Autodesk Inventor part; units mm, degrees
ref_plane "YZ Plane" through (0, 0, 0) normal (1, 0, 0) x (0, 1, 0)
ref_plane "XZ Plane" through (0, 0, 0) normal (0, 1, 0) x (-1, 0, 0)
ref_plane "XY Plane" through (0, 0, 0) normal (0, 0, 1) x (1, 0, 0)
sketch "스케치1" plane through (0, 0, 0) normal (0, 0, 1) x (1, 0, 0)
  line L0 (-103.5, -63) -> (-103.5, 58)
  line L1 (-98.5, -63) -> (-103.5, -63)
  line L2 (-98.5, 58) -> (-98.5, -63)
  line L3 (98.5, 58) -> (-98.5, 58)
  line L4 (98.5, -63) -> (98.5, 58)
  line L5 (103.5, -63) -> (98.5, -63)
  line L6 (103.5, 58) -> (103.5, -63)
  arc A0 (103.5, 58) -> (98.5, 63) centre (98.5, 58) ccw
  line L7 (-98.5, 63) -> (98.5, 63)
  arc A1 (-98.5, 63) -> (-103.5, 58) centre (-98.5, 58) ccw
  line L8 (-98.5, -63) -> (98.5, -63)
  point P0 (0, 0)
extrude "돌출1" add sketch "스케치1" along normal blind 5
sketch "스케치2" plane through (0, 0, 5) normal (0, 0, 1) x (1, 0, 0)
  line L0 (-91.5, 58) -> (91.5, 58)
  line L1 (98.5, 51) -> (98.5, -46)
  line L2 (91.5, -53) -> (-91.5, -53)
  line L3 (-98.5, -46) -> (-98.5, 51)
  line L4 (98.5, 63) -> (-98.5, 63)
  arc A0 (-98.5, 63) -> (-103.5, 58) centre (-98.5, 58) ccw
  line L5 (-103.5, 58) -> (-103.5, -63)
  line L6 (-103.5, -63) -> (103.5, -63)
  line L7 (103.5, -63) -> (103.5, 58)
  arc A1 (103.5, 58) -> (98.5, 63) centre (98.5, 58) ccw
  arc A2 (-91.5, 58) -> (-98.5, 51) centre (-91.5, 51) ccw
  arc A3 (-98.5, -46) -> (-91.5, -53) centre (-91.5, -46) ccw
  arc A4 (91.5, -53) -> (98.5, -46) centre (91.5, -46) ccw
  arc A5 (98.5, 51) -> (91.5, 58) centre (91.5, 51) ccw
  point P0 (0, 0)
  point P1 (98.5, -53)
  point P2 (98.5, 58)
  point P3 (-98.5, -53)
  point P4 (0, 58)
  dimension "d2" = 197
  dimension "d3" = 111
  dimension "d4" = 207
  dimension "d5" = 126
  dimension "d6" = 103.5
  dimension "d7" = 5
  dimension "d8" = 7
extrude "돌출2" cut sketch "스케치2" against normal blind 0.9 contours L0 A5 L1 A4 L2 A3 L3 A2
sketch "스케치3" plane through (0, 0, 4.1) normal (0, 0, 1) x (1, 0, 0)
  line L0 (-82.25, 51.379) -> (83.95, 51.379)
  line L1 (83.95, 51.379) -> (83.95, -49.221)
  line L2 (83.95, -49.221) -> (-82.25, -49.221)
  line L3 (-82.25, -49.221) -> (-82.25, 51.379)
  line L4 (91.5, -53) -> (-91.5, -53)
  arc A0 (91.5, -53) -> (98.5, -46) centre (91.5, -46) ccw
  line L5 (98.5, 51) -> (98.5, -46)
  arc A1 (98.5, 51) -> (91.5, 58) centre (91.5, 51) ccw
  line L6 (-91.5, 58) -> (91.5, 58)
  arc A2 (-91.5, 58) -> (-98.5, 51) centre (-91.5, 51) ccw
  line L7 (-98.5, -46) -> (-98.5, 51)
  arc A3 (-98.5, -46) -> (-91.5, -53) centre (-91.5, -46) ccw
  point P0 (0, 0)
  dimension "d11" = 166.2
  dimension "d12" = 100.6
  dimension "d13" = 14.55
  dimension "d14" = 6.621
sketch "스케치4" plane through (0, 0, 0) normal (0, 0, -1) x (-1, 0, 0)
  line L0 (-98.5, 63) -> (98.5, 63)
  arc A0 (-98.5, 63) -> (-103.5, 58) centre (-98.5, 58) ccw
  line L1 (-103.5, -63) -> (-103.5, 58)
  line L2 (103.5, -63) -> (-103.5, -63)
  line L3 (103.5, 58) -> (103.5, -63)
  arc A1 (103.5, 58) -> (98.5, 63) centre (98.5, 58) ccw
  line L4 (98.5, 58) -> (-98.5, 58)
  line L5 (-98.5, 58) -> (-98.5, -58)
  line L6 (-98.5, -58) -> (98.5, -58)
  line L7 (98.5, -58) -> (98.5, 58)
  point P0 (0, 0)
  dimension "d17" = 5
extrude "돌출4" add sketch "스케치4" along normal blind 1.303 contours L7 L6 L5 L4
extrude "돌출5" cut sketch "스케치3" against normal blind 4.403 contours L0 L1 L2 L3
sketch "스케치6" plane through (0, 0, 4.1) normal (0, 0, 1) x (1, 0, 0)
  line L0 (-93.55, 51) -> (-82.246, 51)
  line L1 (-82.246, 51) -> (-82.246, -46)
  line L2 (-82.246, -46) -> (-93.55, -46)
  line L3 (-93.55, -46) -> (-93.55, 51)
  line L4 (83.95, 51.379) -> (83.95, -49.221)
  line L5 (83.95, -49.221) -> (-82.25, -49.221)
  line L6 (-82.25, -49.221) -> (-82.25, 51.379)
  line L7 (-82.25, 51.379) -> (83.95, 51.379)
  line L8 (91.5, -53) -> (-91.5, -53)
  arc A0 (91.5, -53) -> (98.5, -46) centre (91.5, -46) ccw
  line L9 (98.5, 51) -> (98.5, -46)
  arc A1 (98.5, 51) -> (91.5, 58) centre (91.5, 51) ccw
  line L10 (-91.5, 58) -> (91.5, 58)
  arc A2 (-91.5, 58) -> (-98.5, 51) centre (-91.5, 51) ccw
  line L11 (-98.5, -46) -> (-98.5, 51)
  arc A3 (-98.5, -46) -> (-91.5, -53) centre (-91.5, -46) ccw
  point P0 (0, 0)
  point P1 (-82.25, -46)
  point P2 (-82.25, 51)
  dimension "d22" = 11.304
  dimension "d23" = 97
  dimension "d24" = 4.95
  dimension "d25" = 7
extrude "돌출6" cut sketch "스케치6" against normal blind 0.6 contours L0 L6 L2 L3
sketch "스케치8" plane through (0, 0, -0.303) normal (0, 0, 1) x (1, 0, 0)
  line L0 (-51.5745, 50.756) -> (51.5745, 50.756)
  line L1 (51.5745, 50.756) -> (51.5745, -45.244)
  line L2 (51.5745, -45.244) -> (-51.5745, -45.244)
  line L3 (-51.5745, -45.244) -> (-51.5745, 50.756)
  line L4 (83.95, -49.221) -> (-82.25, -49.221)
  line L5 (83.95, 51.379) -> (83.95, -49.221)
  line L6 (-82.25, 51.379) -> (83.95, 51.379)
  line L7 (-82.25, -49.221) -> (-82.25, 51.379)
  arc A0 (91.5, -53) -> (98.5, -46) centre (91.5, -46) ccw
  line L8 (91.5, -53) -> (-91.5, -53)
  arc A1 (-98.5, -46) -> (-91.5, -53) centre (-91.5, -46) ccw
  line L9 (-98.5, -46) -> (-98.5, 51)
  arc A2 (-91.5, 58) -> (-98.5, 51) centre (-91.5, 51) ccw
  line L10 (-91.5, 58) -> (91.5, 58)
  arc A3 (98.5, 51) -> (91.5, 58) centre (91.5, 51) ccw
  line L11 (98.5, 51) -> (98.5, -46)
  line L12 (98.5, 63) -> (-98.5, 63)
  arc A4 (-98.5, 63) -> (-103.5, 58) centre (-98.5, 58) ccw
  line L13 (-103.5, 58) -> (-103.5, -63)
  line L14 (-103.5, -63) -> (103.5, -63)
  line L15 (103.5, -63) -> (103.5, 58)
  arc A5 (103.5, 58) -> (98.5, 63) centre (98.5, 58) ccw
  line L16 (-69.326, 40.57) -> (-54.826, 40.57)
  line L17 (-54.826, 40.57) -> (-54.826, 32.57)
  line L18 (-54.826, 32.57) -> (-69.326, 32.57)
  line L19 (-69.326, 32.57) -> (-69.326, 40.57)
  line L20 (-69.326, -25.08) -> (-54.826, -25.08)
  line L21 (-54.826, -25.08) -> (-54.826, -33.08)
  line L22 (-54.826, -33.08) -> (-69.326, -33.08)
  line L23 (-69.326, -33.08) -> (-69.326, -25.08)
  line L24 (56.95, 40.57) -> (71.45, 40.57)
  line L25 (71.45, 40.57) -> (71.45, 32.57)
  line L26 (71.45, 32.57) -> (56.95, 32.57)
  line L27 (56.95, 32.57) -> (56.95, 40.57)
  line L28 (56.95, -25.08) -> (71.45, -25.08)
  line L29 (71.45, -25.08) -> (71.45, -33.08)
  line L30 (71.45, -33.08) -> (56.95, -33.08)
  line L31 (56.95, -33.08) -> (56.95, -25.08)
  line L32 (91.5, -53) -> (-91.5, -53)
  arc A6 (91.5, -53) -> (98.5, -46) centre (91.5, -46) ccw
  line L33 (98.5, 51) -> (98.5, -46)
  arc A7 (98.5, 51) -> (91.5, 58) centre (91.5, 51) ccw
  line L34 (-91.5, 58) -> (91.5, 58)
  arc A8 (-91.5, 58) -> (-98.5, 51) centre (-91.5, 51) ccw
  line L35 (-98.5, -46) -> (-98.5, 51)
  arc A9 (-98.5, -46) -> (-91.5, -53) centre (-91.5, -46) ccw
  line L36 (-82.25, -46) -> (-93.55, -46)
  line L37 (-93.55, -46) -> (-93.55, 51)
  line L38 (-93.55, 51) -> (-82.25, 51)
  line L39 (-82.25, 51) -> (-82.25, 51.379)
  line L40 (-82.25, 51.379) -> (83.95, 51.379)
  line L41 (83.95, 51.379) -> (83.95, -49.221)
  line L42 (83.95, -49.221) -> (-82.25, -49.221)
  line L43 (-82.25, -49.221) -> (-82.25, -46)
  point P0 (0, 0)
  point P1 (0, 50.756)
  point P2 (-62.076, -25.069)
  point P3 (-61.0015, 31.581)
  point P4 (-51.5745, 2.756)
  point P5 (50.5, 51.379)
  point P6 (-50.5, 51.379)
  point P7 (-54.826, -29.08)
  point P8 (-54.826, 36.57)
  point P9 (64.2, 40.57)
  point P10 (-62.076, 40.57)
  point P11 (-69.326, -29.08)
  point P12 (-69.326, 36.57)
  dimension "d41" = 96
  dimension "d46" = 197
  dimension "d47" = 98.5
  dimension "d49" = 28.825
  dimension "d53" = 14.5
  dimension "d54" = 8
  dimension "d55" = 14.5
  dimension "d56" = 8
  dimension "d57" = 14.5
  dimension "d58" = 8
  dimension "d59" = 14.5
  dimension "d60" = 8
  dimension "d61" = 27.05
  dimension "d62" = 17.43
  dimension "d63" = 126.276
  dimension "d64" = 65.65
extrude "돌출8" cut sketch "스케치8" against normal blind 2.5 contours L0 L1 L2 L3 | L16 L17 L18 L19 | L20 L21 L22 L23 | L24 L25 L26 L27 | L28 L29 L30 L31
properties part number "AASTRC Top case cover_3D 인쇄"
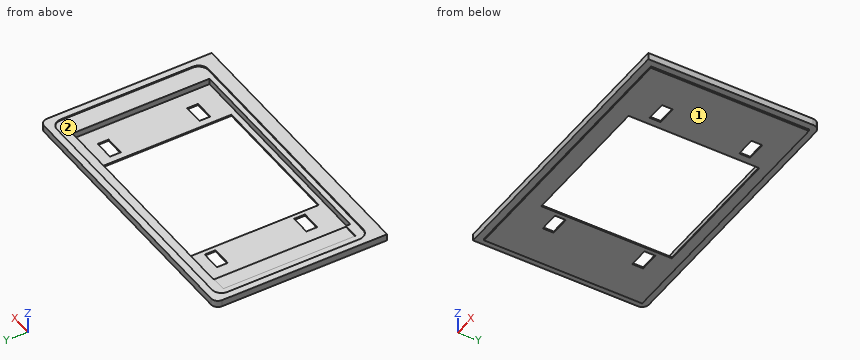
Geometry check sheet. Reference: the model listing, model coordinates, mm. Face numbers are marked on the shaded views. A direction names the side the tool comes from. Give positions to 0.01 mm unless a question says otherwise; leave off trailing zeros. Loops run counter-clockwise (first coordinate to the right, second up) from the corner with the lowest first, then second, coordinate; pieces in that order, holes last. Notation, with made-up numbers: (37.5, 74.5) -> (93.5, 74.5) arc R29 ccw to (93.5, 97.5) -> close; hole circle Ø9 at (15, 55). An arc over 180 degrees is marked (long way). Answer in a Markdown table with one row per item. Add a question column.
1) Cross-section at B-B on y = 7. Record the boundary of the cut face in (x, z), and give its area (3 significant figures).
2) Gauge pin test, flat ends, axial feed: P1, Ø0.5, axis at y = 35, z = -0.5, coming from the -X side; P2, Ø10, axis at x = 61.5, y = 18.5, coming from the +Z side; P3, Ø0.5, axis at y = -28, z = -1, coming from the +X side. Record the tip position at first contact, or that the pin passes through.
3) Set-up check for the marked faces 1 and 2: record each of +Z, -Z, +X, -X, +Y, -Y from which the full face is reachable in a straight line by a thin tool's end or side.
4) Cross-section at D-D on x = 12. Record the boundary of the cut face in (y, z).
5) Material ranges on probe 1 along Y at (x, z) = (-45, 0.75); probe 2 along Y at (x, z) = (-32, -0.25); probe 3 along X at (y, z) = (23, -0.5), recorded low to high. Write a range as from..to.
6) Cross-section at A-A on x = 67.5. Record the boundary of the cut face in (y, z), and give its area (3 significant figures).
7) Cross-section at C-C on z = 2.5. Record the boundary of the cut face in (x, y).
Outcome:
| question | item | result |
|---|---|---|
| 1 | outline | (-103.5, 0) -> (-98.5, 0) -> (-98.5, -1.3) -> (-51.57, -1.3) -> (-51.57, -0.3) -> (-82.25, -0.3) -> (-82.25, 3.5) -> (-93.55, 3.5) -> (-93.55, 4.1) -> (-98.5, 4.1) -> (-98.5, 5) -> (-103.5, 5) -> close; (51.57, -1.3) -> (98.5, -1.3) -> (98.5, 0) -> (103.5, 0) -> (103.5, 5) -> (98.5, 5) -> (98.5, 4.1) -> (83.95, 4.1) -> (83.95, -0.3) -> (51.57, -0.3) -> close |
| 1 | area | 273 mm^2 |
| 2 | P1 | stops at x = -98.5 |
| 2 | P2 | stops at z = -0.3 |
| 2 | P3 | stops at x = 98.5 |
| 3 | face 1 | -Z, +X, -X, +Y, -Y |
| 3 | face 2 | +Z |
| 4 | outline | (-63, 0) -> (-58, 0) -> (-58, -1.3) -> (-45.24, -1.3) -> (-45.24, -0.3) -> (-49.22, -0.3) -> (-49.22, 4.1) -> (-53, 4.1) -> (-53, 5) -> (-63, 5) -> close; (50.76, -1.3) -> (58, -1.3) -> (58, 0) -> (63, 0) -> (63, 5) -> (58, 5) -> (58, 4.1) -> (51.38, 4.1) -> (51.38, -0.3) -> (50.76, -0.3) -> close |
| 5 | probe 1 | y = -63..-49.22, 51.38..63 |
| 5 | probe 2 | y = -58..-49.22, 51.38..58 |
| 5 | probe 3 | x = -98.5..-51.57, 51.57..98.5 |
| 6 | outline | (-63, 0) -> (-58, 0) -> (-58, -1.3) -> (-33.08, -1.3) -> (-33.08, -0.3) -> (-49.22, -0.3) -> (-49.22, 4.1) -> (-53, 4.1) -> (-53, 5) -> (-63, 5) -> close; (-25.08, -1.3) -> (32.57, -1.3) -> (32.57, -0.3) -> (-25.08, -0.3) -> close; (40.57, -1.3) -> (58, -1.3) -> (58, 0) -> (63, 0) -> (63, 5) -> (58, 5) -> (58, 4.1) -> (51.38, 4.1) -> (51.38, -0.3) -> (40.57, -0.3) -> close |
| 6 | area | 222 mm^2 |
| 7 | outline | (-103.5, -63) -> (103.5, -63) -> (103.5, 58) arc R5 ccw to (98.5, 63) -> (-98.5, 63) arc R5 ccw to (-103.5, 58) -> close; hole (-82.25, -49.22) -> (83.95, -49.22) -> (83.95, 51.38) -> (-82.25, 51.38) -> close |
